Can you work these out from the model? Positions are in its coordinate system, mm. A direction names the side the tool comes from. Give positions to 0.01 mm unless a question says otherwise; leave off trailing zeros. Write each loop counter-clockwise with the first axis right and the second up, starting at its lowest first coordinate (ties: lowest second). Pieces come first, ordered by that corner, then holes.
from build123d import *

# Parameters (mm, degrees)
F1_DEPTH = 18
F2_R     = 2


with BuildPart() as f1:
    # F0 (on Front) → F1 (new body)
    with BuildSketch(Plane.XZ):
        with BuildLine():
            Line((54.3322916932, 202.7708730905), (0, 0))
            Line((0, 0), (35.456227742, 0))
            Line((35.456227742, 0), (111.5254217963, 163.130913087))
            ThreePointArc((111.5254217963, 163.130913087), (129.9758307308, 184.1695722906), (156.8408111482, 192))
            Line((156.8408111482, 192), (343.1591888518, 192))
            ThreePointArc((343.1591888518, 192), (370.0241692692, 184.1695722906), (388.4745782037, 163.130913087))
            Line((388.4745782037, 163.130913087), (464.543772258, 0))
            Line((464.543772258, 0), (500, 0))
            Line((500, 0), (434.0056960838, 258.2940952255))
            ThreePointArc((434.0056960838, 258.2940952255), (432.2198740974, 260.9667667015), (429.1760669523, 262))
            Line((429.1760669523, 262), (371.6265428539, 262))
            Line((371.6265428539, 262), (344.9233630828, 262))
            ThreePointArc((344.9233630828, 262), (341.3878291768, 260.5355339059), (339.9233630828, 257))
            Line((339.9233630828, 257), (339.9233630828, 242))
            Line((339.9233630828, 242), (139.9233630828, 242))
            Line((139.9233630828, 242), (139.9233630828, 257))
            ThreePointArc((139.9233630828, 257), (138.4588969887, 260.5355339059), (134.9233630828, 262))
            Line((134.9233630828, 262), (128.3734571461, 262))
            ThreePointArc((128.3734571461, 262), (81.6327118159, 244.5364204466), (54.3322916932, 202.7708730905))
        make_face()
    extrude(amount=F1_DEPTH)

    # F2
    f2_edges = [f1.edges().sort_by_distance(p)[0] for p in [
        (339.923363, -18, 249.5),
        (239.923363, -18, 242),
        (139.923363, -18, 249.5),
        (138.458897, -18, 260.535534),
        (131.64841, -18, 262),
        (81.632712, -18, 244.53642),
        (27.166146, -18, 101.385437),
        (17.728114, -18, 0),
        (73.490825, -18, 81.565457),
        (129.975831, -18, 184.169572),
        (250, -18, 192),
        (370.024169, -18, 184.169572),
        (426.509175, -18, 81.565457),
        (482.271886, -18, 0),
        (467.002848, -18, 129.147048),
        (432.219874, -18, 260.966767),
        (387.049715, -18, 262),
        (341.387829, -18, 260.535534),
        (339.923363, 0, 249.5),
        (239.923363, 0, 242),
        (139.923363, 0, 249.5),
        (138.458897, 0, 260.535534),
        (131.64841, 0, 262),
        (81.632712, 0, 244.53642),
        (27.166146, 0, 101.385437),
        (17.728114, 0, 0),
        (73.490825, 0, 81.565457),
        (129.975831, 0, 184.169572),
        (250, 0, 192),
        (370.024169, 0, 184.169572),
        (426.509175, 0, 81.565457),
        (482.271886, 0, 0),
        (467.002848, 0, 129.147048),
        (432.219874, 0, 260.966767),
        (387.049715, 0, 262),
        (341.387829, 0, 260.535534),
    ]]
    fillet(f2_edges, radius=F2_R)


solid = f1.part
(1) Will these pins go through, and if not, where does the flat tip stop? P1, Ø4, axis at x = 194.5, y = -10, coming from the +Z side; P2, Ø1, axis at y = -6.5, z = 29.5, coming from the -X side; P3, Ø4, axis at y = -9.5, z = 247, coming from the +X side.
Returned:
P1: stops at z = 242
P2: stops at x = 7.77
P3: stops at x = 437.4
(2) Imagine slicing it at B-B, the plane x = 271. Write out the boundary of the cut face in (y, z).
Returned:
outline: (-18, 194) arc R2 ccw to (-16, 192) - (-2, 192) arc R2 ccw to (0, 194) - (0, 240) arc R2 ccw to (-2, 242) - (-16, 242) arc R2 ccw to (-18, 240) - close
(3) If we mould it in two halves opening along X, with no side actions, what happens to faces 5 (the face through (427.56, -17.4, 80.66)), 6 (the face through (17, -9, 0)), 7 (the face through (27.546, -8.902, 102.805))? For each: +X half, -X half, draft (parallel to the pull), parting line (faces both ways), or undercut.
Returned:
face 5: undercut
face 6: draft
face 7: -X half
(4) For faces 1 (the face through (73.506, -17.399, 82.948)), 2 (the face through (73.506, -0.601, 82.948)), 3 (the face through (249, -9, 192)), 4 (the face through (139.923, -9, 249)), which set-ups out of +Z, -Z, +X, -X, +Y, -Y let a thin tool reach every point of the face, with its end or its side?
Returned:
face 1: -Z, -Y
face 2: -Z, +Y
face 3: -Z, +Y, -Y
face 4: +Z, +Y, -Y
(5) Imagine slicing it at A-A, the plane y = -8.75. Write out the boundary of the cut face in (x, z), plus the area to 3 significant figures.
Returned:
outline: (0, 0) - (35.46, 0) - (111.53, 163.13) arc R50 cw to (156.84, 192) - (343.16, 192) arc R50 cw to (388.47, 163.13) - (464.54, 0) - (500, 0) - (434.01, 258.29) arc R5 ccw to (429.18, 262) - (344.92, 262) arc R5 ccw to (339.92, 257) - (339.92, 242) - (139.92, 242) - (139.92, 257) arc R5 ccw to (134.92, 262) - (128.37, 262) arc R80 ccw to (54.33, 202.77) - close
area: 43,500 mm2
(6) If I drill on L1, parallel to X at y = -11, z = 32; L2, parallel to X at y = -1.75, z = 243; L3, parallel to Z at x = 174.5, y = -2.75, over which ranges is the centre line in solid material (lowest first)?
Returned:
L1: x = 8.57 to 50.38, 449.62 to 491.82
L2: x = 79.79 to 139.91, 339.94 to 437.9
L3: z = 192 to 242
